Part model, mm, in its own coordinate system. A direction names the side the tool comes from. Give positions to 0.01 mm unless a question says otherwise; leave off trailing zeros. Order: outer loops, then holes, each group sorted by start corner. A loop starts at its lowest first (then second) coordinate and runs counter-clockwise, first axis right, second up.
from build123d import *

# Parameters (mm, degrees)
F0_W     = 25.4
F0_H     = 25.4
F1_DEPTH = 127
F2_W     = 50.8
F2_H     = 50.8
F3_DEPTH = 101.6
F4_W     = 76.2
F4_H     = 76.2
F5_DEPTH = 76.2
F6_W     = 101.6
F6_H     = 101.6
F7_DEPTH = 50.8
F8_W     = 127
F8_H     = 127
F9_DEPTH = 25.4
F10_R    = 5.08


with BuildPart() as f1:
    # F0 (on Top) → F1 (new body)
    with BuildSketch(Plane.XY):
        Rectangle(F0_W, F0_H)
    extrude(amount=F1_DEPTH)

    # F2 (on Top) → F3 (join)
    with BuildSketch(Plane.XY):
        Rectangle(F2_W, F2_H)
    extrude(amount=F3_DEPTH)

    # F4 (on Top) → F5 (join)
    with BuildSketch(Plane.XY):
        Rectangle(F4_W, F4_H)
    extrude(amount=F5_DEPTH)

    # F6 (on Top) → F7 (join)
    with BuildSketch(Plane.XY):
        Rectangle(F6_W, F6_H)
    extrude(amount=F7_DEPTH)

    # F8 (on Top) → F9 (join)
    with BuildSketch(Plane.XY):
        Rectangle(F8_W, F8_H)
    extrude(amount=F9_DEPTH)

    # F10
    f10_edges = [f1.edges().sort_by_distance(p)[0] for p in [
        (0, -12.7, 127),
        (0, -25.4, 101.6),
        (0, -38.1, 76.2),
        (0, -50.8, 50.8),
        (0, -63.5, 25.4),
        (12.7, 0, 127),
        (0, 12.7, 127),
        (-12.7, 0, 127),
        (25.4, 0, 101.6),
        (0, 25.4, 101.6),
        (-25.4, 0, 101.6),
        (38.1, 0, 76.2),
        (0, 38.1, 76.2),
        (-38.1, 0, 76.2),
        (-50.8, 0, 50.8),
        (-63.5, 0, 25.4),
        (50.8, 0, 50.8),
        (63.5, 0, 25.4),
        (0, 50.8, 50.8),
        (0, 63.5, 25.4),
    ]]
    fillet(f10_edges, radius=F10_R)


solid = f1.part
Item 1: Band-saw the part on C-C on z = 36.5. List the corners of the cut face in (x, y), plus the area to 3 significant figures.
Item 2: Band-saw the part on A-A on y = 16.5. List the corners of the cut face in (x, z).
Item 3: Drill centre lines: probe 1 along Y at (x, z) = (3.5, 119); probe 2 along Z at (x, y) = (-31, 46); probe 3 along Y at (x, z) = (21, 77.5). Where is each one in solid material? Low to high.
Item 4: Which spindle directions (+Z, -Z, +X, -X, +Y, -Y) get a long thin tool onto all of the face, cutting with end or side? Do faces 1 (the face through (-1, -38.1, 61)), 2 (the face through (0, 12.7, 112)), 3 (the face through (-38.1, -1, 61)). Say none if no direction does.
Item 5: Drop flat-ended pins along their axis: P1, Ø8, axis at y = -45.5, z = 31.5, coming from the -X side; P2, Ø16.5, axis at y = 3.5, z = 81.5, coming from the +X side; P3, Ø6, axis at x = 5.5, z = 108.5, coming from the -Y side. Give the stop position or say it passes through.
Item 6: Band-saw the part on D-D on x = -43.5. List the corners of the cut face in (y, z), plus the area to 3 significant figures.
Working result:
1. outline: (-50.8, -50.8) - (50.8, -50.8) - (50.8, 50.8) - (-50.8, 50.8) - close
1. area: 10,300 mm2
2. outline: (-63.5, 0) - (63.5, 0) - (63.5, 20.32) arc R5.08 ccw to (58.42, 25.4) - (50.8, 25.4) - (50.8, 45.72) arc R5.08 ccw to (45.72, 50.8) - (38.1, 50.8) - (38.1, 71.12) arc R5.08 ccw to (33.02, 76.2) - (25.4, 76.2) - (25.4, 96.52) arc R5.08 ccw to (20.32, 101.6) - (-20.32, 101.6) arc R5.08 ccw to (-25.4, 96.52) - (-25.4, 76.2) - (-33.02, 76.2) arc R5.08 ccw to (-38.1, 71.12) - (-38.1, 50.8) - (-45.72, 50.8) arc R5.08 ccw to (-50.8, 45.72) - (-50.8, 25.4) - (-58.42, 25.4) arc R5.08 ccw to (-63.5, 20.32) - close
3. probe 1: y = -12.7 to 12.7
3. probe 2: z = 0 to 50.79
3. probe 3: y = -25.4 to 25.4
4. face 1: +Z, +X, -X, -Y
4. face 2: +Z, +X, -X, +Y
4. face 3: +Z, -X, +Y, -Y
5. P1: stops at x = -50.8
5. P2: stops at x = 37.63
5. P3: stops at y = -12.7
6. outline: (-63.5, 0) - (63.5, 0) - (63.5, 20.32) arc R5.08 ccw to (58.42, 25.4) - (50.8, 25.4) - (50.8, 45.72) arc R5.08 ccw to (45.72, 50.8) - (-45.72, 50.8) arc R5.08 ccw to (-50.8, 45.72) - (-50.8, 25.4) - (-58.42, 25.4) arc R5.08 ccw to (-63.5, 20.32) - close
6. area: 5,780 mm2
